from build123d import *

# Parameters (mm, degrees)
CYLINDER_R     = 16
CYLINDER_DEPTH = 3.4
BOX002_W       = 50
BOX002_H       = 29
BOX002_DEPTH   = 4
BOX001_W       = 58
BOX001_H       = 24
BOX001_DEPTH   = 30
BOX_W          = 54
BOX_H          = 36
BOX_DEPTH      = 9


with BuildPart() as lens_hole:
    # Cylinder → Cylinder (new body)
    with BuildSketch(Plane.XY.offset(-1.7)):
        Circle(CYLINDER_R)
    extrude(amount=CYLINDER_DEPTH)


with BuildPart() as inner_lens_extraction_cube:
    # Box002 → Box002 (new body)
    with BuildSketch(Plane(origin=(-11, -14.5, -2), x_dir=(1, 0, 0), z_dir=(0, 0, 1))):
        with Locations((25, 14.5)):
            Rectangle(BOX002_W, BOX002_H)
    extrude(amount=BOX002_DEPTH)


with BuildPart() as holder_cut_fusion:
    # Box001 → Box001 (new body)
    with BuildSketch(Plane(origin=(-10, -12, -15), x_dir=(1, 0, 0), z_dir=(0, 0, 1))):
        with Locations((29, 12)):
            Rectangle(BOX001_W, BOX001_H)
    extrude(amount=BOX001_DEPTH)

    # Fusion: union lens hole, inner lens extraction cube
    add(lens_hole.part)
    add(inner_lens_extraction_cube.part)


with BuildPart() as holder_cut:
    # Box → Box (new body)
    with BuildSketch(Plane(origin=(-16, -18, -4.5), x_dir=(1, 0, 0), z_dir=(0, 0, 1))):
        with Locations((27, 18)):
            Rectangle(BOX_W, BOX_H)
    extrude(amount=BOX_DEPTH)

    # Cut: cut holder cut fusion
    add(holder_cut_fusion.part, mode=Mode.SUBTRACT)


solid = holder_cut.part
Design review of the part built by this model. Coordinates are the model's own, in mm. A direction names the side the tool comes from. Coordinates: 2 decimals unless noted, no trailing zeros. Order: outer loops, then holes, each group sorted by start corner. A loop starts at its lowest first (then second) coordinate and runs counter-clockwise, first axis right, second up. Notation, with made-up numbers: (31.25, 40.5) - (60.25, 40.5) arc R15 cw to (60.25, 58.5) - close; hole circle Ø5 at (59, 25). An arc over 180 degrees is marked (long way). Put each result on its own line as item: value.
1) Take a section at D-D, the plane z = -3.5. Give the boundary of the cut face in (x, y).
Response values:
outline: (-16, -18) - (38, -18) - (38, -12) - (-10, -12) - (-10, 12) - (38, 12) - (38, 18) - (-16, 18) - close
2) Wall thickness on L1, parallel to Y at x = 7, z = 1; L2, parallel to Y at x = -9, z = 2.25; L3, parallel to Z at x = -10.5, y = -6: over which ranges is each line inside the solid? List them lowest first. Write a range as from..to.
Response values:
L1: y = -18..-14.5, 14.5..18
L2: y = -18..-12, 12..18
L3: z = -4.5..-2, 2..4.5
3) Tool access review of faces 1 (the face through (14, 12, 3)), 2 (the face through (10, -13, -2)), 3 (the face through (11, -18, 0)), 4 (the face through (0, 16, 0)): name each direction out of +Z, -Z, +X, -X, +Y, -Y from which nothing blocks a thin tool from reaching the whole face with its end or side.
Response values:
face 1: +Z, -Z, +X
face 2: +X
face 3: +Z, -Z, +X, -X, -Y
face 4: none
4) Insertion check: P1, Ø3, axis at y = 2, z = 3.5, coming from the +X side; P2, Ø10, axis at x = 10, y = -7.5, coming from the +Z side; P3, Ø2, axis at y = -8, z = 0, coming from the +X side. Each pin has a flat end and moves straight along its axis. Give the tip position at first contact, or say it passes through.
Response values:
P1: stops at x = -10
P2: stops at z = 4.5
P3: stops at x = -13.23
5) Take a section at C-C, the plane y = -2.5. Give the boundary of the cut face in (x, z), and give its area (3 significant figures).
Response values:
outline: (-16, -4.5) - (-10, -4.5) - (-10, -2) - (-11, -2) - (-11, -1.7) - (-15.8, -1.7) - (-15.8, 1.7) - (-11, 1.7) - (-11, 2) - (-10, 2) - (-10, 4.5) - (-16, 4.5) - close
area: 33.7 mm²
6) The part is to be moulded in two halves that separate along X. For faces 5 (the face through (19, 14.5, 0)), 6 (the face through (0, 15, 1.7)), 7 (the face through (-16, 0, 2)), say which applies: released by +X, released by -X, zero draft, split by the parting line, or undercut.
Response values:
face 5: zero draft
face 6: undercut
face 7: released by -X
7) Take a section at B-B, the plane x = 7.5. Give the boundary of the cut face in (y, z).
Response values:
outline: (-18, -4.5) - (-12, -4.5) - (-12, -2) - (-14.5, -2) - (-14.5, 2) - (-12, 2) - (-12, 4.5) - (-18, 4.5) - close; (12, -4.5) - (18, -4.5) - (18, 4.5) - (12, 4.5) - (12, 2) - (14.5, 2) - (14.5, -2) - (12, -2) - close
